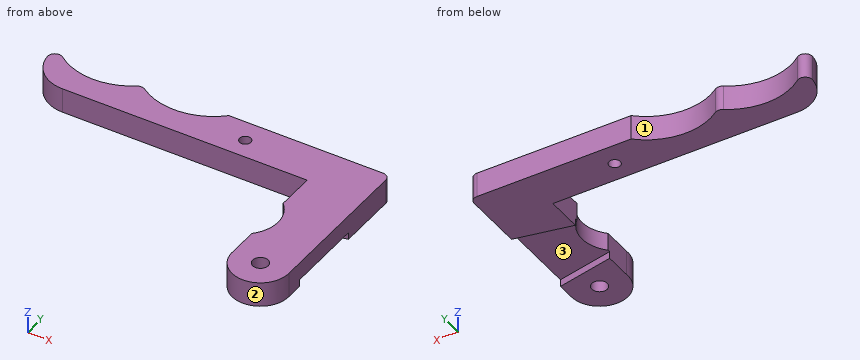
from build123d import *

# Parameters (mm, degrees)
SKETCH_R     = 2.2
SKETCH_R_2   = 1.6
PAD_DEPTH    = 7
POCKET_DEPTH = 2


with BuildPart() as part:
    # Sketch → Pad (new body)
    with BuildSketch(Plane.XY):
        with BuildLine():
            Line((-37.186391, 18), (31.875645, 18))
            Line((31.875645, 18), (31.875645, 7.116152))
            ThreePointArc((31.875645, -7.116152), (34.849951, 0), (31.875645, 7.116152))
            Line((31.875645, -7.116152), (31.875645, -15.359342))
            ThreePointArc((31.875645, -15.359342), (39.629949, -23.996974), (47.847419, -15.798736))
            Line((47.847419, -15.798736), (47.847419, 28))
            ThreePointArc((47.847419, 28), (47.261632, 29.414214), (45.847419, 30))
            Line((45.847419, 30), (2.298191, 30))
            ThreePointArc((-20.439447, 28.328622), (-8.772276, 25.105501), (2.298191, 30))
            ThreePointArc((-20.439447, 28.328622), (-21.583605, 28.69212), (-22.729772, 28.335007))
            ThreePointArc((-43.934553, 28.826581), (-33.412258, 25.125755), (-22.729772, 28.335007))
            ThreePointArc((-43.934553, 28.826581), (-46.120226, 28.987251), (-47.140964, 27.047901))
            ThreePointArc((-47.140964, 27.047901), (-43.912423, 20.599967), (-37.186391, 18))
        make_face()
        with Locations((39.849951, -16)):
            Circle(SKETCH_R, mode=Mode.SUBTRACT)
        with Locations((10.846568, 23.709484)):
            Circle(SKETCH_R_2, mode=Mode.SUBTRACT)
    extrude(amount=PAD_DEPTH)

    # Sketch001 → Pocket (cut)
    with BuildSketch(Plane(origin=(0, 0, 0), x_dir=(1, 0, 0), z_dir=(0, 0, -1))):
        Polygon((8.880411, 3), (52.827053, 12.125178), (52.827053, -12.125178), (8.880411, -3), align=None)
    extrude(amount=-POCKET_DEPTH, mode=Mode.SUBTRACT)


solid = part.part
Geometry: final body of the model. Coordinates: model frame, mm. Face numbers are marked on the shaded views. Coordinates: 2 decimals unless noted, no trailing zeros. Order: outer loops, then holes, each group sorted by start corner. A loop starts at its lowest first (then second) coordinate and runs counter-clockwise, first axis right, second up. Notation, with made-up numbers: (50, 87) - (83, 87) arc R14 ccw to (83, 113) - close; hole circle Ø9 at (19.5, 74). An arc over 180 degrees is marked (long way). Use one line per item in the form item = value.
1) Section A-A (z = 3.25). Return loops of the section in (x, y) (3 decimals), then the cut area to 3 significant figures.
Solutions:
outline = (-47.141, 27.048) arc R10 ccw to (-37.186, 18) - (31.876, 18) - (31.876, 7.116) arc R10 cw to (31.876, -7.116) - (31.876, -15.359) arc R8 ccw (long way) to (47.847, -15.799) - (47.847, 28) arc R2 ccw to (45.847, 30) - (2.298, 30) arc R18 cw to (-20.439, 28.329) arc R2 ccw to (-22.73, 28.335) arc R18 cw to (-43.935, 28.827) arc R2 ccw to start; hole circle Ø3.2 at (10.847, 23.709); hole circle Ø4.4 at (39.85, -16)
area = 1,540 mm^2
2) Section B-B (x = 19). Return loops of the section in (y, z), then the cut area to 3 significant figures.
Solutions:
outline = (18, 0) - (30, 0) - (30, 7) - (18, 7) - close
area = 84.0 mm^2
3) Pin query (flat end, axial travel): pin 1 (2 mm diameter, centred on y = -1.5, z = 2, fed in from +X); pin 2 (8 mm diameter, centred on x = 38, y = 3, fed in from -Z); pin 3 (4 mm diameter, centred on x = 16, z = 6, fed in from -Y). Return the tip coordinate at first contact, or that it passes through.
Solutions:
pin_1 = 47.85
pin_2 = 2
pin_3 = 18
4) Mould query, pull axis X, two halves, no side actions, for the marked faces 1, 2 and 3. Classes: +X half, -X half, draft (parallel to the pull), parting line (faces both ways), or undercut.
Solutions:
face_1 = undercut
face_2 = parting line
face_3 = draft
5) Ray query, L1, parallel to Y at x = 29.5, z = 4; L2, parallel to X at y = -10, z = 6; L3, parallel to Y at x = -7, z = 1.5. Return the intervals inside material, ascending.
Solutions:
L1 = 18 to 30
L2 = 31.88 to 47.85
L3 = 18 to 25.32
6) Section C-C (y = 1). Return loops of the section in (x, z).
Solutions:
outline = (34.8, 2) - (47.85, 2) - (47.85, 7) - (34.8, 7) - close
